Design review of the part shown in the three views and the two pictorial views. Dimensions are in mm from the part's minimum x, y and z. A direction names the side the tool comes from. Give positions to 0.01 mm unless a question says otherwise; leave off trailing zeros. Order: outer loops, then holes, each group sorted by start corner. A loop starts at its lowest first (then second) coordinate and runs counter-clockwise, first axis right, second up. Notation, with made-up numbers: (21, -16) -> (76, -16) arc R14 ccw to (76, -7) -> close; hole circle Ø3 at (38.25, 45). An arc over 180 degrees is marked (long way). Use one line per item in the form item = value.
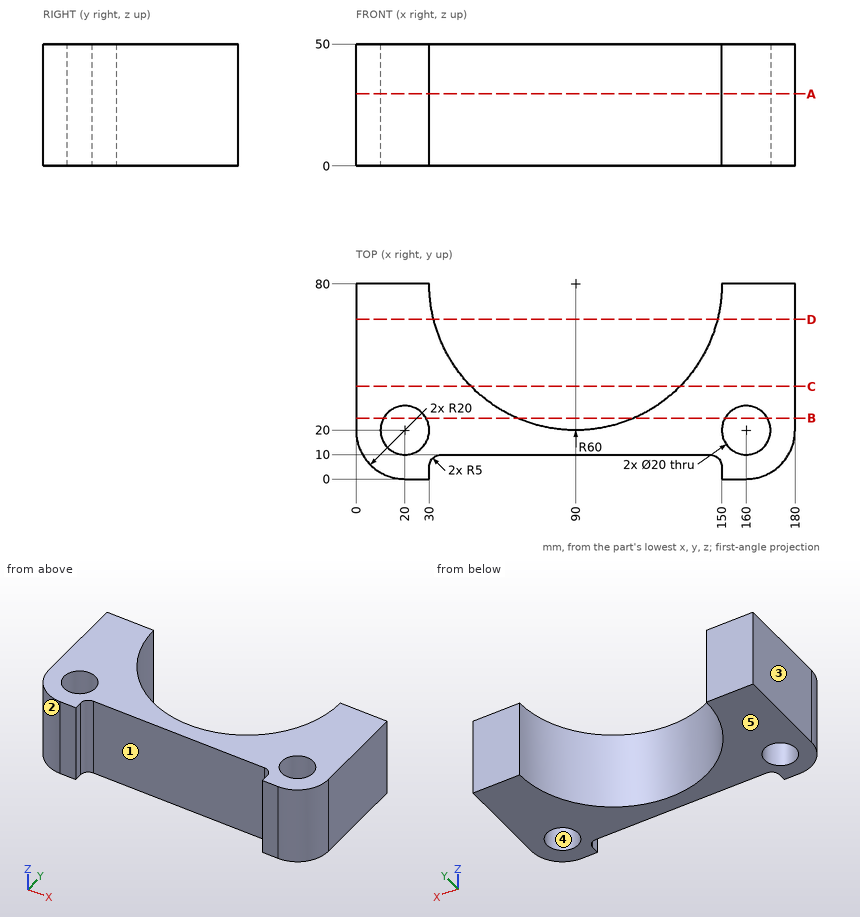
1. Add section A-A on z = 29.5. Give the boundary of the cut face in (x, y), then the cut area to 3 significant figures.
Values:
outline = (0, 20) arc R20 ccw to (20, 0) -> (30, 0) -> (30, 5) arc R5 cw to (35, 10) -> (145, 10) arc R5 cw to (150, 5) -> (150, 0) -> (160, 0) arc R20 ccw to (180, 20) -> (180, 80) -> (150, 80) arc R60 cw to (30, 80) -> (0, 80) -> close; hole circle Ø20 at (20, 20); hole circle Ø20 at (160, 20)
area = 6,760 mm^2
2. Add section C-C on y = 38. Give the boundary of the cut face in (x, z), then the cut area to 3 significant figures.
Values:
outline = (0, 0) -> (47.15, 0) -> (47.15, 50) -> (0, 50) -> close; (132.85, 0) -> (180, 0) -> (180, 50) -> (132.85, 50) -> close
area = 4,720 mm^2
3. The part is to be moulded in two halves that separate along X. For the marked faces 3, 4 and 5, say which applies: +X half, -X half, draft (parallel to the pull), parting line (faces both ways), or undercut.
Values:
face_3 = -X half
face_4 = undercut
face_5 = draft
4. Add section D-D on y = 65.5. Give the boundary of the cut face in (x, z), then the cut area to 3 significant figures.
Values:
outline = (0, 0) -> (31.78, 0) -> (31.78, 50) -> (0, 50) -> close; (148.22, 0) -> (180, 0) -> (180, 50) -> (148.22, 50) -> close
area = 3,180 mm^2
5. Add section B-B on y = 25. Give the boundary of the cut face in (x, z), then the cut area to 3 significant figures.
Values:
outline = (0, 0) -> (11.34, 0) -> (11.34, 50) -> (0, 50) -> close; (28.66, 0) -> (66.02, 0) -> (66.02, 50) -> (28.66, 50) -> close; (113.98, 0) -> (151.34, 0) -> (151.34, 50) -> (113.98, 50) -> close; (168.66, 0) -> (180, 0) -> (180, 50) -> (168.66, 50) -> close
area = 4,870 mm^2
6. Tool access review of the marked faces 1 and 2: name each direction out of +Z, -Z, +X, -X, +Y, -Y from which nothing blocks a thin tool from reaching the whole face with its end or side.
Values:
face_1 = +Z, -Z, -Y
face_2 = +Z, -Z, -X, -Y
7. For pin 1 Ø2 at (y, z) = (9, 43) entering from -X; pin 2 Ø1 at (y, z) = (10, 23.5) entering from -X; pin 3 Ø2 at (x, z) = (91.5, 30.5) entering from +Y; pin 4 Ø18 at (x, y) = (20, 20) entering from -Z, all flat-tipped, find the tip position at first contact; note any pin that passes through.
Values:
pin_1 = 2.68
pin_2 = 2.4
pin_3 = 20.05
pin_4 = through
8. For L1, parallel to Y at x = 160, z = 12; L2, parallel to X at y = 56, z = 2; L3, parallel to X at y = 25, z = 4.5, list the stretches that pass through material, from the lowest coordinate up.
Values:
L1 = 0 to 10, 30 to 80
L2 = 0 to 35.01, 144.99 to 180
L3 = 0 to 11.34, 28.66 to 66.02, 113.98 to 151.34, 168.66 to 180
